from build123d import *

# Parameters (mm, degrees)
SKETCH1_R           = 3.556
BOSS_EXTRUDE1_DEPTH = 9.398


with BuildPart() as part:
    # Sketch1 → Boss-Extrude1 (new, symmetric)
    with BuildSketch(Plane(origin=(0, 0, 0), x_dir=(1, 0, 0), z_dir=(0, 1, 0))):
        with BuildLine():
            Line((0, 8.255), (61.468, 8.255))
            ThreePointArc((61.468, 8.255), (69.723, 0), (61.468, -8.255))
            Line((61.468, -8.255), (0, -8.255))
            ThreePointArc((0, -8.255), (-8.255, 0), (0, 8.255))
        make_face()
        with Locations(Location((0, 0, 0), (0, 0, 270))):
            Circle(SKETCH1_R, mode=Mode.SUBTRACT)
        with Locations(Location((25.5524, 0, 0), (0, 0, 270))):
            Circle(SKETCH1_R, mode=Mode.SUBTRACT)
        with Locations(Location((61.468, 0, 0), (0, 0, 270))):
            Circle(SKETCH1_R, mode=Mode.SUBTRACT)
    extrude(amount=BOSS_EXTRUDE1_DEPTH, both=True)


solid = part.part
For this review, take the finished solid that the model builds, in its own axes (mm). Give positions to 0.01 mm unless a question says otherwise; leave off trailing zeros. Loops run counter-clockwise (first coordinate to the right, second up) from the corner with the lowest first, then second, coordinate; pieces in that order, holes last.
Item 1: Take a section at A-A, the plane z = 0. State the section outline as (x, y) points (3 decimals), and give its area (3 significant figures).
Item 2: Insertion check: pin 1 (5.5 mm diameter, centred on x = 61.468, z = 0, fed in from +Y); pin 2 (6 mm diameter, centred on y = -3, z = 4, fed in from -X); pin 3 (3 mm diameter, centred on y = -7, z = -3, fed in from -X); pin 4 (1 mm diameter, centred on y = -0.5, z = 4.5, fed in from +X). Each pin has a flat end and moves straight along its axis. Give the tip position at first contact, or say it passes through.
Item 3: Draft analysis for pull direction X (two halves, no side actions). For faces 1 (the cylindrical face through (69.72, 0.13, -0.18)), 2 (the cylindrical face through (64.994, -0.132, -0.463)), 3 (the flat face through (31, 9.398, 0)), 4 (the cylindrical face through (-8.253, 0.132, 0.182)), state which applies: +X half, -X half, draft (parallel to the pull), parting line (faces both ways), or undercut.
Item 4: For line 1 along X through (y, z) = (1, 0) (3 decimals); line 2 along X through (y, z) = (3.25, -3); line 3 along Z through (x, y) = (59, 0.75) (3 decimals), list the stretches that pass through material, from the lowest coordinate up.
Item 5: Take a section at B-B, the plane x = 27. State the section outline as (y, z) points (3 decimals).
Item 6: Take a section at C-C, the plane y = -5.25. State the section outline as (x, z) points (3 decimals), and give its area (3 significant figures).
Calculated:
1. outline: (-8.255, -9.398) - (-3.556, -9.398) - (-3.556, 9.398) - (-8.255, 9.398) - close; (3.556, -9.398) - (21.996, -9.398) - (21.996, 9.398) - (3.556, 9.398) - close; (29.108, -9.398) - (57.912, -9.398) - (57.912, 9.398) - (29.108, 9.398) - close; (65.024, -9.398) - (69.723, -9.398) - (69.723, 9.398) - (65.024, 9.398) - close
1. area: 1,060 mm2
2. pin 1: passes through
2. pin 2: stops at x = -8.19
2. pin 3: stops at x = -8.12
2. pin 4: stops at x = 68.69
3. face 1: +X half
3. face 2: undercut
3. face 3: draft
3. face 4: -X half
4. line 1: x = -8.255 to -3.556, 3.556 to 21.996, 29.108 to 57.912, 65.024 to 69.723
4. line 2: x = -7.69 to -1.91, 1.91 to 23.64, 27.46 to 59.56, 63.38 to 69.16
4. line 3: z = -8.255 to -2.56, 2.56 to 8.255
5. outline: (-9.398, -8.255) - (9.398, -8.255) - (9.398, -3.248) - (-9.398, -3.248) - close; (-9.398, 3.248) - (9.398, 3.248) - (9.398, 8.255) - (-9.398, 8.255) - close
6. outline: (0, -8.255) - (61.468, -8.255) arc R8.255 ccw to (61.468, 8.255) - (0, 8.255) arc R8.255 ccw to start; hole circle Ø7.112 at (0, 0); hole circle Ø7.112 at (25.552, 0); hole circle Ø7.112 at (61.468, 0)
6. area: 1,110 mm2
